For this review, take the finished solid that the model builds, in its own axes (mm). Give positions to 0.01 mm unless a question says otherwise; leave off trailing zeros. Loops run counter-clockwise (first coordinate to the right, second up) from the corner with the lowest first, then second, coordinate; pieces in that order, holes last. Notation, with made-up numbers: (61.5, -8.75) -> (100.5, -8.75) arc R32 ccw to (100.5, 26.25) -> close; hole circle Ø1 at (27.5, 17.5). An arc over 180 degrees is marked (long way). Answer as CSV lines item,"result". Start each with the question number.
Item 1: For L1, parallel to X at y = -14.5, z = 4; L2, parallel to Z at x = 4, y = -17; L3, parallel to Z at x = -5, y = -2, list the stretches that pass through material, from the lowest coordinate up. Write a range as from..to.
Item 2: Add section D-D on x = 14.5. State the section outline as (y, z) points.
Item 3: Add section A-A on z = 10. State the section outline as (x, y) points, plus the area to 3 significant figures.
Item 4: Clearance check with flat-ended pins moving along their axes: P1, Ø4, axis at y = -8, z = 7, coming from the -X side; P2, Ø5, axis at y = -2.5, z = -37, coming from the -X side; P3, Ø1.5, axis at x = 42, y = -14, coming from the -Z side; P4, Ø23, axis at x = 0, z = 0, coming from the +Y side. State where each tip first meets the part, or that it passes through.
Item 5: Add section C-C on x = 32.5. State the section outline as (y, z) points.
Item 6: The part is to be moulded in two halves that separate along X. For faces 1 (the face through (-2.75, -9.39, -12.4)), 2 (the face through (-5, 0, -13)), say which applies: +X half, -X half, draft (parallel to the pull), parting line (faces both ways), or undercut.
Item 7: Add section B-B on y = -8. State how many separate pieces and enclosed holes the cut face has, plus the area to 3 significant figures.
```python
from build123d import *

# Parameters (mm, degrees)
F0_R     = 12.7
F1_DEPTH = 19.05


with BuildPart() as f1:
    # F0 (on Front) → F1 (new body)
    with BuildSketch(Plane.XZ):
        with BuildLine():
            Line((12.23147, 52.190307), (6.35, 52.190307))
            ThreePointArc((6.35, 52.190307), (0, 45.840307), (-6.35, 52.190307))
            Line((-6.35, 52.190307), (-13.16853, 52.190307))
            ThreePointArc((-13.16853, 52.190307), (-24.185423, 24.077807), (-52.602746, 13.872888))
            Line((-52.602746, 13.872888), (-52.602746, 6.35))
            ThreePointArc((-52.602746, 6.35), (-48.112618, 4.490128), (-46.252746, 0))
            ThreePointArc((-46.252746, 0), (-48.112618, -4.490128), (-52.602746, -6.35))
            Line((-52.602746, -6.35), (-52.602746, -12.031119))
            ThreePointArc((-52.602746, -12.031119), (-23.888564, -22.029354), (-12.7, -50.300982))
            Line((-12.7, -50.300982), (-6.35, -50.300982))
            ThreePointArc((-6.35, -50.300982), (0, -43.950982), (6.35, -50.300982))
            Line((6.35, -50.300982), (12.7, -50.300982))
            ThreePointArc((12.7, -50.300982), (23.267131, -22.677459), (50.825791, -11.942305))
            Line((50.825791, -11.942305), (50.825791, -6.35))
            ThreePointArc((50.825791, -6.35), (44.475791, 0), (50.825791, 6.35))
            Line((50.825791, 6.35), (50.825791, 13.234786))
            ThreePointArc((50.825791, 13.234786), (22.719563, 23.985158), (12.23147, 52.190307))
        make_face()
        Circle(F0_R, mode=Mode.SUBTRACT)
        with BuildLine():
            ThreePointArc((0, 58.540307), (4.490128, 56.680435), (6.35, 52.190307))
            Line((6.35, 52.190307), (12.23147, 52.190307))
            ThreePointArc((12.23147, 52.190307), (8.675876, 61.003356), (0, 64.881661))
            Line((0, 64.881661), (0, 58.540307))
        make_face()
        with BuildLine():
            ThreePointArc((-6.35, 52.190307), (-4.490128, 56.680435), (0, 58.540307))
            Line((0, 58.540307), (0, 64.881661))
            ThreePointArc((0, 64.881661), (-9.281579, 61.334713), (-13.16853, 52.190307))
            Line((-13.16853, 52.190307), (-6.35, 52.190307))
        make_face()
        with BuildLine():
            ThreePointArc((65.188185, 0), (61.110783, 9.985633), (50.825791, 13.234786))
            Line((50.825791, 13.234786), (50.825791, 6.35))
            ThreePointArc((50.825791, 6.35), (55.315919, 4.490128), (57.175791, 0))
            Line((57.175791, 0), (65.188185, 0))
        make_face()
        with BuildLine():
            Line((-52.602746, 6.35), (-52.602746, 13.872888))
            ThreePointArc((-52.602746, 13.872888), (-61.916345, 9.656853), (-65.272424, 0))
            Line((-65.272424, 0), (-58.952746, 0))
            ThreePointArc((-58.952746, 0), (-57.092874, 4.490128), (-52.602746, 6.35))
        make_face()
        with BuildLine():
            ThreePointArc((50.825791, -11.942305), (60.624398, -9.118977), (65.188185, 0))
            Line((65.188185, 0), (57.175791, 0))
            ThreePointArc((57.175791, 0), (55.315919, -4.490128), (50.825791, -6.35))
            Line((50.825791, -6.35), (50.825791, -11.942305))
        make_face()
        with BuildLine():
            Line((-58.952746, 0), (-65.272424, 0))
            ThreePointArc((-65.272424, 0), (-61.271138, -8.472967), (-52.602746, -12.031119))
            Line((-52.602746, -12.031119), (-52.602746, -6.35))
            ThreePointArc((-52.602746, -6.35), (-57.092874, -4.490128), (-58.952746, 0))
        make_face()
        with BuildLine():
            ThreePointArc((0, -63.000982), (8.980256, -59.281238), (12.7, -50.300982))
            Line((12.7, -50.300982), (6.35, -50.300982))
            ThreePointArc((6.35, -50.300982), (4.490128, -54.79111), (0, -56.650982))
            Line((0, -56.650982), (0, -63.000982))
        make_face()
        with BuildLine():
            Line((-6.35, -50.300982), (-12.7, -50.300982))
            ThreePointArc((-12.7, -50.300982), (-8.980256, -59.281238), (0, -63.000982))
            Line((0, -63.000982), (0, -56.650982))
            ThreePointArc((0, -56.650982), (-4.490128, -54.79111), (-6.35, -50.300982))
        make_face()
    extrude(amount=F1_DEPTH)


solid = f1.part
```
Computed values:
1,L1,"-64.93..-57.53, -47.67..-12.05, 12.05..45.89, 55.76..64.75"
1,L2,"-62.35..-55.23, -45.37..-12.05, 12.05..47.26, 57.12..64.08"
1,L3,"-61.98..-54.22, -46.39..-11.67, 11.67..48.28, 56.1..64.05"
2,outline,"(-19.05, -36.95) -> (0, -36.95) -> (0, 36.78) -> (-19.05, 36.78) -> close"
3,outline,"(-61.59, -19.05) -> (-7.83, -19.05) -> (-7.83, 0) -> (-61.59, 0) -> close; (7.83, -19.05) -> (61.1, -19.05) -> (61.1, 0) -> (7.83, 0) -> close"
3,area,"2,040 mm²"
4,P1,"x = -64.65"
4,P2,"x = -15.39"
4,P3,"z = -12.77"
4,P4,"through"
5,outline,"(-19.05, -15.93) -> (0, -15.93) -> (0, 16.94) -> (-19.05, 16.94) -> close"
6,face 1,"undercut"
6,face 2,"draft"
7,separate pieces,"1"
7,enclosed holes,"5"
7,area,"5,760 mm²"
